from build123d import *

# Parameters (mm, degrees)
SKETCH1_W                       = 80
SKETCH1_H                       = 70
BOSS_EXTRUDE1_DEPTH             = 35.5
CUT_EXTRUDE1_REACH              = 72
SKETCH2_W                       = 59
SKETCH2_H                       = 24.5
SKETCH6_R                       = 27.5
CUT_EXTRUDE3_DEPTH              = 5.5
M4X0_7_TAPPED_HOLE1_D           = 3.3
M4X0_7_TAPPED_HOLE1_DEPTH       = 5.5
FILLET2_R                       = 2
SKETCH9_W                       = 80
SKETCH9_H                       = 70
CUT_EXTRUDE5_DEPTH              = 5.5
TAP_DRILL_FOR_M3X0_5_TAP1_D     = 2.5
TAP_DRILL_FOR_M3X0_5_TAP1_DEPTH = 15
TAP_DRILL_FOR_M3X0_5_TAP1_TIP   = 0.751075774
FILLET5_R                       = 2
FILLET6_R                       = 2
FILLET7_R                       = 4.5
FILLET8_R                       = 4.5
TAP_DRILL_FOR_M3X0_5_TAP2_D     = 2.5
TAP_DRILL_FOR_M3X0_5_TAP2_DEPTH = 15
TAP_DRILL_FOR_M3X0_5_TAP2_TIP   = 0.751075774


with BuildPart() as part:
    # Sketch1 → Boss-Extrude1 (new body)
    with BuildSketch(Plane(origin=(0, 0, 0), x_dir=(1, 0, 0), z_dir=(0, 1, 0))):
        with Locations((-2.631253278, 2.602774632)):
            Rectangle(SKETCH1_W, SKETCH1_H)
    extrude(amount=BOSS_EXTRUDE1_DEPTH)

    # Sketch2 → Cut-Extrude1 (cut, up to next)
    with BuildSketch(Plane.XY.offset(32.397225368), mode=Mode.PRIVATE) as cut_extrude1_sk1:
        with Locations((-2.631253278, 17.75)):
            Rectangle(SKETCH2_W, SKETCH2_H)
    cut_extrude1_tool1 = extrude(cut_extrude1_sk1.sketch, amount=-CUT_EXTRUDE1_REACH, mode=Mode.PRIVATE) & part.part
    add(cut_extrude1_tool1.solids().sort_by_distance((-2.631253, 17.75, 32.397225))[0], mode=Mode.SUBTRACT)

    # Sketch6 → Cut-Extrude3 (cut)
    with BuildSketch(Plane.XZ):
        with Locations(Location((-2.631253278, -2.602774632, 0), (0, 0, 270))):  # turned: the seam where the file's is
            Circle(SKETCH6_R)
    extrude(amount=-CUT_EXTRUDE3_DEPTH, mode=Mode.SUBTRACT)

    # M4x0.7 Tapped Hole1
    with Locations(Plane(origin=(22.368746722, 0, 22.397225368), x_dir=(0, 0, -1), z_dir=(0, -1, 0))):
        with Locations((0, 0), (50, 0), (50, -50), (0, -50)):
            Hole(M4X0_7_TAPPED_HOLE1_D / 2, depth=M4X0_7_TAPPED_HOLE1_DEPTH)

    # Fillet2
    fillet2_edges = [part.edges().sort_by_distance(p)[0] for p in [
        (-2.631253278, 0, 24.897225368),
    ]]
    fillet(fillet2_edges, radius=FILLET2_R)

    # Sketch9 → Cut-Extrude5 (cut)
    with BuildSketch(Plane(origin=(0, 35.5, 0), x_dir=(-1, 0, 0), z_dir=(0, 1, 0))):
        with Locations((2.631253278, -2.602774632)):
            Rectangle(SKETCH9_W, SKETCH9_H)
    extrude(amount=-CUT_EXTRUDE5_DEPTH, mode=Mode.SUBTRACT)

    # Tap Drill for M3x0.5 Tap1
    with Locations(Plane(origin=(-37.381253278, 30, -32.352774632), x_dir=(0, 0, 1), z_dir=(0, 1, 0))):
        with Locations((0, 0), (29.75, 0), (59.5, 0), (0, 69.5), (29.5, 69.5), (59.5, 69.5)):
            Hole(TAP_DRILL_FOR_M3X0_5_TAP1_D / 2, depth=TAP_DRILL_FOR_M3X0_5_TAP1_DEPTH)
            with Locations((0, 0, -(TAP_DRILL_FOR_M3X0_5_TAP1_DEPTH + TAP_DRILL_FOR_M3X0_5_TAP1_TIP / 2))):  # 118° drill point
                Cone(0, TAP_DRILL_FOR_M3X0_5_TAP1_D / 2, TAP_DRILL_FOR_M3X0_5_TAP1_TIP, mode=Mode.SUBTRACT)

    # Fillet5
    fillet5_edges = [part.edges().sort_by_distance(p)[0] for p in [
        (-42.631253278, 15, 32.397225368),
    ]]
    fillet(fillet5_edges, radius=FILLET5_R)

    # Fillet6
    fillet6_edges = [part.edges().sort_by_distance(p)[0] for p in [
        (-42.631253278, 15, -37.602774632),
    ]]
    fillet(fillet6_edges, radius=FILLET6_R)

    # Fillet7
    fillet7_edges = [part.edges().sort_by_distance(p)[0] for p in [
        (-32.131253278, 17.75, 32.397225368),
        (-2.631253278, 5.5, 32.397225368),
        (26.868746722, 17.75, 32.397225368),
    ]]
    fillet(fillet7_edges, radius=FILLET7_R)

    # Fillet8
    fillet8_edges = [part.edges().sort_by_distance(p)[0] for p in [
        (-2.631253278, 5.5, -37.602774632),
        (-32.131253278, 17.75, -37.602774632),
        (26.868746722, 17.75, -37.602774632),
    ]]
    fillet(fillet8_edges, radius=FILLET8_R)

    # Tap Drill for M3x0.5 Tap2
    with Locations(Plane(origin=(32.618746722, 0, 12.397225368), x_dir=(0, 0, -1), z_dir=(0, -1, 0))):
        with Locations((0, 0), (30, 0), (0, -70.5), (30, -70.5)):
            Hole(TAP_DRILL_FOR_M3X0_5_TAP2_D / 2, depth=TAP_DRILL_FOR_M3X0_5_TAP2_DEPTH)
            with Locations((0, 0, -(TAP_DRILL_FOR_M3X0_5_TAP2_DEPTH + TAP_DRILL_FOR_M3X0_5_TAP2_TIP / 2))):  # 118° drill point
                Cone(0, TAP_DRILL_FOR_M3X0_5_TAP2_D / 2, TAP_DRILL_FOR_M3X0_5_TAP2_TIP, mode=Mode.SUBTRACT)


solid = part.part
Source: CAD feature listing. Evaluate the final solid. Frame: model axes, mm. A direction names the side the tool comes from. Round coordinates to 2 decimals unless told otherwise and drop trailing zeros. Loops run counter-clockwise (first coordinate to the right, second up) from the corner with the lowest first, then second, coordinate; pieces in that order, holes last. Notation, with made-up numbers: M 68,-38 L 122,-38 A29 ccw 122,-18 Z; hole C 44,-8.75 d3. An arc over 180 degrees is marked long. Return JSON: item names as keys, results as strings. Group by question number.
1. Mould query, pull axis X, two halves, no side actions, for faces 5 (the face through (32.334, 14.379, 27.119)), 6 (the face through (6.9, 0.5, 32.397)), 7 (the face through (-42.631, 15, -2)). Classes: released by +X, released by -X, zero draft, split by the parting line, or undercut.
2. Section query A-A on y = 19.25. Output: boundary loops of the cut face in (x, z).
3. Section query B-B on y = 12.5. Output: boundary loops of the cut face in (x, z), and give its area (3 significant figures).
4. Material intervals for line 1 along X through (y, z) = (8, 21.5); line 2 along X through (y, z) = (2.5, -3.5); line 3 along Y through (x, z) = (26, 20.5), sorted ascending. Write a range as from..to.
5. Section query C-C on z = -27.5. State how many separate pieces and enclosed holes the cut face has, and give its area (3 significant figures).
6. Reachability of faces 1 (the face through (-36.14, 22.4, -2.44)), 2 (the face through (-32.131, 18, -2)), 3 (the face through (32.67, 7.6, -18.85)), 4 (the face through (-2.16, 4.15, 31.11)) from +Z, -Z, +X, -X, +Y, -Y: full face, straight path, thin tool, end or side. Return the list, or none.
7. Pin query (flat end, axial travel): pin 1 (3 mm diameter, centred on x = 32.62, z = 12.4, fed in from -Y); pin 2 (1.5 mm diameter, centred on x = 32.12, z = 27.15, fed in from +Y); pin 3 (6 mm diameter, centred on x = 19.5, y = 7.5, fed in from -Z); pin 4 (1 mm diameter, centred on x = -20.5, y = 3.5, fed in from -Z). Return the tip coordinate at first contact, or that it passes through.
Checks:
{
 "1": {"face 5": "undercut", "face 6": "zero draft", "face 7": "released by -X"},
 "2": {"outline": "M -42.63,-35.6 A2 ccw -40.63,-37.6 L -36.63,-37.6 A4.5 ccw -32.13,-33.1 L -32.13,27.9 A4.5 ccw -36.63,32.4 L -40.63,32.4 A2 ccw -42.63,30.4 Z; M 26.87,-33.1 A4.5 ccw 31.37,-37.6 L 37.37,-37.6 L 37.37,32.4 L 31.37,32.4 A4.5 ccw 26.87,27.9 Z; hole C -37.38,-32.35 d2.5; hole C -37.38,-2.6 d2.5; hole C -37.38,27.15 d2.5; hole C 32.12,-32.35 d2.5; hole C 32.12,-2.85 d2.5; hole C 32.12,27.15 d2.5"},
 "3": {"outline": "M -42.63,-35.6 A2 ccw -40.63,-37.6 L -36.63,-37.6 A4.5 ccw -32.13,-33.1 L -32.13,27.9 A4.5 ccw -36.63,32.4 L -40.63,32.4 A2 ccw -42.63,30.4 Z; M 26.87,-33.1 A4.5 ccw 31.37,-37.6 L 37.37,-37.6 L 37.37,32.4 L 31.37,32.4 A4.5 ccw 26.87,27.9 Z; hole C -37.88,-17.6 d2.5; hole C -37.88,12.4 d2.5; hole C 32.62,-17.6 d2.5; hole C 32.62,12.4 d2.5", "area": "1,430 mm²"},
 "4": {"line 1": "x = -42.63..-32.13, 26.87..37.37", "line 2": "x = -42.63..-30.12, 24.85..37.37", "line 3": "y = 0..5.5"},
 "5": {"separate pieces": "4", "enclosed holes": "0", "area": "786 mm²"},
 "6": {"face 1": "+Y", "face 2": "+Z, -Z, +Y", "face 3": "-Y", "face 4": "+Z, +Y"},
 "7": {"pin 1": "stops at y = 0", "pin 2": "stops at y = 14.7", "pin 3": "stops at z = -35.93", "pin 4": "stops at z = -37.13"}
}
